Read the model definition and answer for the solid it produces. Units are mm, in the model's axes. Face numbers are marked on the shaded views. A direction names the side the tool comes from. Coordinates: 2 decimals unless noted, no trailing zeros.
from build123d import *

# Parameters (mm, degrees)
BOSS_EXTRUDE1_DEPTH      = 4.7625
BOSS_EXTRUDE1_DEPTH_BACK = 4.7625
SKETCH11_R               = 3.3274
SKETCH11_R_2             = 2.413
CUT_EXTRUDE1_START       = 3.095625
SKETCH12_R               = 3.3274
SKETCH12_R_2             = 3.175
CUT_EXTRUDE1_DEPTH       = 1.666875
CHAMFER2_SIZE            = 0.3048
CHAMFER2_SIZE2           = 0.527929086
EXTRUDE4_DEPTH           = 7.695116711
EXTRUDE4_DEPTH_BACK      = 7.695116711
SKETCH8_W                = 0.9525
SKETCH8_H                = 7.14375


# Read off the part's stored shape, not the designer's step: Cut-Extrude3, Cut-Extrude10
with BuildPart() as part:
    # Sketch11 → Boss-Extrude1 (new, two sides: drawn at the far end of the back side and taken through both)
    with BuildSketch(Plane(origin=(0, 0, 0), x_dir=(1, 0, 0), z_dir=(0, 1, 0)).offset(-BOSS_EXTRUDE1_DEPTH_BACK)):
        with Locations(Location((0, 0, 0), (0, 0, 90))):
            Circle(SKETCH11_R)
        with Locations(Location((0, 0, 0), (0, 0, 90))):
            Circle(SKETCH11_R_2, mode=Mode.SUBTRACT)
    extrude(amount=BOSS_EXTRUDE1_DEPTH + BOSS_EXTRUDE1_DEPTH_BACK)

    # Sketch12 → Cut-Extrude1 (cut)
    with BuildSketch(Plane(origin=(0, 0, 0), x_dir=(1, 0, 0), z_dir=(0, 1, 0)).offset(CUT_EXTRUDE1_START)):
        with Locations(Location((0, 0, 0), (0, 0, 90))):
            Circle(SKETCH12_R)
        with Locations(Location((0, 0, 0), (0, 0, 270))):
            Circle(SKETCH12_R_2, mode=Mode.SUBTRACT)
    extrude(amount=CUT_EXTRUDE1_DEPTH, mode=Mode.SUBTRACT)

    # Cut-Extrude3 outline → Cut-Extrude3 (revolve, cut)
    with BuildSketch(Plane.XY):
        Polygon((2.413, 4.7625), (2.413, 4.52537515), (2.6543, 4.7625), align=None)
    revolve(axis=Axis((0, 0, 0), (0, 1, 0)), mode=Mode.SUBTRACT)

    # Cut-Extrude10 outline → Cut-Extrude10 (revolve, cut)
    with BuildSketch(Plane.XY):
        Polygon((2.6543, -4.7625), (2.413, -4.52537515), (2.413, -4.7625), align=None)
    revolve(axis=Axis((0, 0, 0), (0, 1, 0)), mode=Mode.SUBTRACT)

    # Chamfer2
    chamfer2_edges = [part.edges().sort_by_distance(p)[0] for p in [
        (0, -4.7625, 3.3274),
    ]]
    chamfer2_side = [part.faces().sort_by_distance(p)[0] for p in [
        (0, -4.7625, 3.233286916),
    ]]
    chamfer(chamfer2_edges, length=CHAMFER2_SIZE, length2=CHAMFER2_SIZE2, reference=chamfer2_side[0])

    # Sketch8 → Extrude4 (cut, two sides: drawn at the far end of the back side and taken through both)
    with BuildSketch(Plane.XY.offset(-EXTRUDE4_DEPTH_BACK)):
        with Locations((0, -1.190625)):
            Rectangle(SKETCH8_W, SKETCH8_H)
    extrude(amount=EXTRUDE4_DEPTH + EXTRUDE4_DEPTH_BACK, mode=Mode.SUBTRACT)


solid = part.part
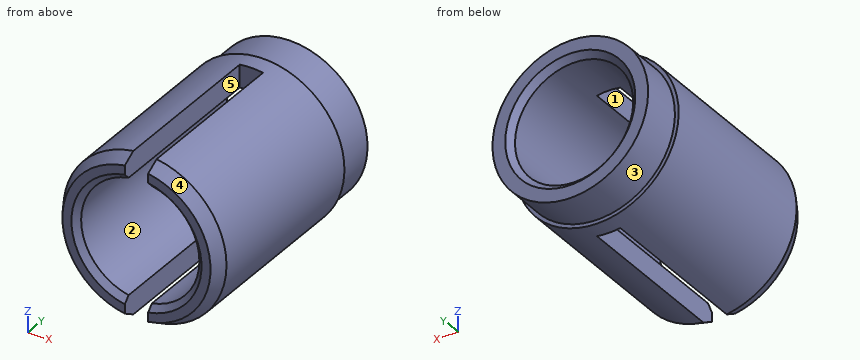
Q1. Straight lines are drawn through the part: L1, parallel to X at y = 0.75, z = 0; L2, parallel to Z at x = 2, y = 3; L3, parallel to X at y = -2, z = -3. For each, find the intervals that lie inside material, in ascending order.
Q2. Which of the six approach directions +Z, -Z, +X, -X, +Y, -Y give full straight-line access (tool end or side, diameter ignored) to the marked faces 1 and 2?
Q3. Determine the mould class of the marked faces 3, 4 and 5 for opening direction X: +X half, -X half, draft (parallel to the pull), parting line (faces both ways), or undercut.
Q4. Each of these flat-tipped pins is pushed along its axis until it touches: P1, Ø0.7, axis at y = -1, z = -2.5, coming from the -X side; P2, Ø0.5, axis at x = 0, z = 3, coming from the -Y side; P3, Ø1, axis at x = 2, y = 0.5, coming from the -Z side. Where does it stop, or does it pass through?
Computed values:
1. L1: x = -3.33 to -2.41, 2.41 to 3.33
1. L2: z = -2.66 to -1.35, 1.35 to 2.66
1. L3: x = -1.44 to -0.48, 0.48 to 1.44
2. face 1: +Z, -Z, -Y
2. face 2: +Y, -Y
3. face 3: parting line
3. face 4: +X half
3. face 5: undercut
4. P1: stops at x = -2.54
4. P2: stops at y = 2.38
4. P3: stops at z = -2.97
